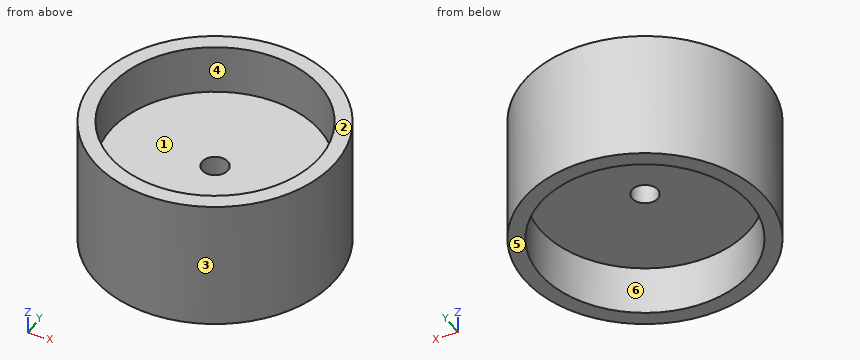
```python
from build123d import *

# Parameters (mm, degrees)
F0_W     = 5.8166
F0_H     = 48.26
F2_R     = 38.6334
F2_R_2   = 4.7625
F3_DEPTH = 5.7912


with BuildPart() as f1:
    # F0 (on Front) → F1 (revolve)
    with BuildSketch(Plane.XZ):
        with Locations((41.5417, 0)):
            Rectangle(F0_W, F0_H)
    revolve(axis=Axis((0, 0, 0), (0, 0, -1)))

    # F2 (on Top) → F3 (join, symmetric)
    with BuildSketch(Plane.XY):
        Circle(F2_R)
        Circle(F2_R_2, mode=Mode.SUBTRACT)
    extrude(amount=F3_DEPTH, both=True)


solid = f1.part
```
Read the model definition and answer for the solid it produces. Units are mm, in the model's axes. Face numbers are marked on the shaded views. A direction names the side the tool comes from. Round coordinates to 2 decimals unless told otherwise and drop trailing zeros. Loops run counter-clockwise (first coordinate to the right, second up) from the corner with the lowest first, then second, coordinate; pieces in that order, holes last. Notation, with made-up numbers: (13.5, 40.25) -> (72.5, 40.25) arc R8 cw to (72.5, 44.25) -> close; hole circle Ø4 at (-5, -27.5). An arc over 180 degrees is marked (long way). One line per item, written item: value.
1) The mould has two halves that part along X. Classify the marked faces 1, 2 and 3: pulls with the +X half, pulls with the -X half, needs draft (parallel to the pull), parting line crosses it, or undercut.
Answer list:
face 1: undercut
face 2: needs draft
face 3: parting line crosses it
2) Flat-ended cylindrical pins translate along their axes: P1, Ø10, axis at x = -4.5, z = 16, coming from the -Y side; P2, Ø8, axis at x = 10, z = -1, coming from the +Y side; P3, Ø10, axis at x = 34, z = 10.5, coming from the -Y side. Find the tip coordinate at first contact, or state that the pin passes through.
Answer list:
P1: stops at y = -44.45
P2: stops at y = 44.04
P3: stops at y = -33.69
3) A cutting plane is placed at A-A (y = 0). Determine the outline of the cut face in (x, z), and give its area (3 significant figures).
Answer list:
outline: (-44.45, -24.13) -> (-38.63, -24.13) -> (-38.63, -5.79) -> (-4.76, -5.79) -> (-4.76, 5.79) -> (-38.63, 5.79) -> (-38.63, 24.13) -> (-44.45, 24.13) -> close; (4.76, -5.79) -> (38.63, -5.79) -> (38.63, -24.13) -> (44.45, -24.13) -> (44.45, 24.13) -> (38.63, 24.13) -> (38.63, 5.79) -> (4.76, 5.79) -> close
area: 1,350 mm²
4) Consider L1, parallel to Y at x = 0, z = 16; L2, parallel to Y at x = 0, z = 0. Determine where each line is inside the solid, lowest interval first. Write a range as [from, to].
Answer list:
L1: y = [-44.45, -38.63], [38.63, 44.45]
L2: y = [-44.45, -4.76], [4.76, 44.45]
5) For the marked faces 4, 5 and 6, determine the directions among +Z, -Z, +X, -X, +Y, -Y from which every point of the face is accessible in a straight line to the end or side of a thin tool.
Answer list:
face 4: +Z
face 5: -Z, +X, -X, +Y, -Y
face 6: -Z
6) A cutting plane is placed at D-D (x = 31). Determine the outline of the cut face in (y, z), and give its area (3 significant figures).
Answer list:
outline: (-31.86, -24.13) -> (-23.06, -24.13) -> (-23.06, -5.79) -> (23.06, -5.79) -> (23.06, -24.13) -> (31.86, -24.13) -> (31.86, 24.13) -> (23.06, 24.13) -> (23.06, 5.79) -> (-23.06, 5.79) -> (-23.06, 24.13) -> (-31.86, 24.13) -> close
area: 1,380 mm²
